```python
from build123d import *

# Parameters (mm, degrees)
F1_DEPTH = 5
F2_W     = 2
F2_H     = 6
F3_DEPTH = 2.5
F4_SIZE  = 1


with BuildPart() as f1:
    # F0 (on Top) → F1 (new body, symmetric)
    with BuildSketch(Plane.XY):
        Polygon((15.3884176859, 5), (9.510565163, 13.0901699437), (0, 16.1803398875), (-9.510565163, 13.0901699437), (-15.3884176859, 5), (-15.3884176859, -5), (-9.510565163, -13.0901699437), (0, -16.1803398875), (9.510565163, -13.0901699437), (15.3884176859, -5), align=None)
        with BuildLine():
            ThreePointArc((1.5198684154, 1.3), (0, -2), (-1.5198684154, 1.3))
            Line((-1.5198684154, 1.3), (1.5198684154, 1.3))
        make_face(mode=Mode.SUBTRACT)
    extrude(amount=F1_DEPTH, both=True)

    # F2 (on Top) → F3 (join, symmetric)
    with BuildSketch(Plane.XY):
        with Locations((16.3884176859, 0)):
            Rectangle(F2_W, F2_H)
        Polygon((15.83088117, 7.7936044933), (12.3041696563, 12.6477064596), (10.6861356675, 11.472135955), (14.2128471813, 6.6180339887), align=None)
        Polygon((8.2264861191, 15.6103169651), (2.5201470213, 17.4644189313), (1.9021130326, 15.5623058987), (7.6084521304, 13.7082039325), align=None)
        Polygon((-2.5201470213, 17.4644189313), (-8.2264861191, 15.6103169651), (-7.6084521304, 13.7082039325), (-1.9021130326, 15.5623058987), align=None)
        Polygon((-12.3041696563, 12.6477064596), (-15.83088117, 7.7936044933), (-14.2128471813, 6.6180339887), (-10.6861356675, 11.472135955), align=None)
        with Locations((-16.3884176859, 0)):
            Rectangle(F2_W, F2_H)
        Polygon((-15.83088117, -7.7936044933), (-12.3041696563, -12.6477064596), (-10.6861356675, -11.472135955), (-14.2128471813, -6.6180339887), align=None)
        Polygon((-8.2264861191, -15.6103169651), (-2.5201470213, -17.4644189313), (-1.9021130326, -15.5623058987), (-7.6084521304, -13.7082039325), align=None)
        Polygon((2.5201470213, -17.4644189313), (8.2264861191, -15.6103169651), (7.6084521304, -13.7082039325), (1.9021130326, -15.5623058987), align=None)
        Polygon((12.3041696563, -12.6477064596), (15.83088117, -7.7936044933), (14.2128471813, -6.6180339887), (10.6861356675, -11.472135955), align=None)
    extrude(amount=F3_DEPTH, both=True)

    # F4
    f4_edges = [f1.edges().sort_by_distance(p)[0] for p in [
        (12.30417, -12.647706, 0),
        (15.830881, -7.793604, 0),
        (17.388418, -3, 0),
        (17.388418, 3, 0),
        (15.830881, 7.793604, 0),
        (12.30417, 12.647706, 0),
        (8.226486, 15.610317, 0),
        (2.520147, 17.464419, 0),
        (-2.520147, 17.464419, 0),
        (-8.226486, 15.610317, 0),
        (-12.30417, 12.647706, 0),
        (-15.830881, 7.793604, 0),
        (-17.388418, 3, 0),
        (-17.388418, -3, 0),
        (-15.830881, -7.793604, 0),
        (-12.30417, -12.647706, 0),
        (-2.520147, -17.464419, 0),
        (-8.226486, -15.610317, 0),
        (8.226486, -15.610317, 0),
        (2.520147, -17.464419, 0),
    ]]
    chamfer(f4_edges, length=F4_SIZE)


solid = f1.part
```
Geometry check sheet. Reference: the model listing, model coordinates, mm. A direction names the side the tool comes from. Give positions to 0.01 mm unless a question says otherwise; leave off trailing zeros. Order: outer loops, then holes, each group sorted by start corner. A loop starts at its lowest first (then second) coordinate and runs counter-clockwise, first axis right, second up.
1. Access from +Z, -Z, +X, -X, +Y, -Y to the whole of each face (thin tool, end or side, straight path). Record for faces 5 (the face through (13, 9, 2.5)), 6 (the face through (16, -3, 0)), 7 (the face through (2.85, 16.84, -0.03)), 8 (the face through (2.85, -16.84, 0.03)), 9 (the face through (-5, 15, -2.5)).
2. Section check C-C, the plane x = -1. Enter the section's corners in (y, z), and give its area (3 significant figures).
3. Release check for a two-part mould opening along X. For faces 1 (the face through (14.051, -10.243, 0.035)), 2 (the face through (11.08, -11.76, 0.04)), 3 (the face through (2.054, -16.031, -0.035)), 4 (the face through (-7.765, 14.19, -0.035)) record: pulls with the +X half, pulls with the -X half, needs draft (parallel to the pull), parting line crosses it, or undercut.
4. Gauge pin test, flat ends, axial feed: pin 1 Ø8 at (x, y) = (12.5, -11.5) entering from -Z; pin 2 Ø1 at (x, y) = (4.5, -16) entering from +Z; pin 3 Ø1 at (x, y) = (6, -15) entering from -Z; pin 4 Ø1.5 at (y, z) = (11.5, -1.5) entering from +X. Record the tip position at first contact, or that the pin passes through.
5. Section check D-D, the plane x = -5.5. Enter the section's corners in (y, z), and give its area (3 significant figures).
6. Section check B-B, the plane y = 0. Enter the section's corners in (x, z), and give its area (3 significant figures).
7. Section check A-A, the plane z = 3. Enter the section's corners in (x, y).
8. Thickness scan on L1, parallel to X at y = 0, z = -0.5; L2, parallel to Y at x = 0, z = -2.5; L3, parallel to Y at x = -14.5, z = -2. Record the ranges inside material, lowest first.
Values follow:
1. face 5: +Z, +X, +Y
1. face 6: +Z, -Z, +X, -Y
1. face 7: +Z, -Z, +Y
1. face 8: +Z, -Z, -Y
1. face 9: -Z, -X, +Y
2. outline: (-15.86, -5) - (-1.73, -5) - (-1.73, 5) - (-15.86, 5) - close; (1.3, -5) - (15.86, -5) - (15.86, 5) - (1.3, 5) - close
2. area: 287 mm2
3. face 1: pulls with the +X half
3. face 2: undercut
3. face 3: undercut
3. face 4: pulls with the -X half
4. pin 1: stops at z = -5
4. pin 2: stops at z = 2.5
4. pin 3: stops at z = -2.5
4. pin 4: stops at x = 13.68
5. outline: (-16.5, -2.5) - (-14.39, -2.5) - (-14.39, -5) - (14.39, -5) - (14.39, -2.5) - (16.5, -2.5) - (16.5, 2.5) - (14.39, 2.5) - (14.39, 5) - (-14.39, 5) - (-14.39, 2.5) - (-16.5, 2.5) - close
5. area: 309 mm2
6. outline: (-17.39, -2.5) - (-15.39, -2.5) - (-15.39, -5) - (-2, -5) - (-2, 5) - (-15.39, 5) - (-15.39, 2.5) - (-17.39, 2.5) - close; (2, -5) - (15.39, -5) - (15.39, -2.5) - (17.39, -2.5) - (17.39, 2.5) - (15.39, 2.5) - (15.39, 5) - (2, 5) - close
6. area: 288 mm2
7. outline: (-15.39, -5) - (-9.51, -13.09) - (0, -16.18) - (9.51, -13.09) - (15.39, -5) - (15.39, 5) - (9.51, 13.09) - (0, 16.18) - (-9.51, 13.09) - (-15.39, 5) - close; hole (-1.52, 1.3) arc R2 ccw (long way) to (1.52, 1.3) - close
8. L1: x = -17.39 to -2, 2 to 17.39
8. L2: y = -16.18 to -2, 1.3 to 16.18
8. L3: y = -9.63 to -6.83, -6.22 to 6.22, 6.83 to 9.63
